from build123d import *

# Parameters (mm, degrees)
F0_W     = 68
F0_H     = 160.5
F1_DEPTH = 10
F2_W     = 46
F2_H     = 17
F3_DEPTH = 25
F4_R     = 5.5
F5_DEPTH = 25
F6_W     = 15
F6_H     = 10
F7_DEPTH = 4
F8_W     = 7
F8_H     = 7
F9_DEPTH = 7


with BuildPart() as f1:
    # F0 (on Front) → F1 (new body)
    with BuildSketch(Plane.XZ):
        with Locations((4.173387, 26.878738)):
            Rectangle(F0_W, F0_H)
    extrude(amount=F1_DEPTH)

    # F2 (on face) → F3 (cut)
    with BuildSketch(Plane.XZ.offset(10)):
        with Locations((-6.826613, 98.628738)):
            Rectangle(F2_W, F2_H)
    extrude(amount=-F3_DEPTH, mode=Mode.SUBTRACT)

    # F4 (on face) → F5 (cut)
    with BuildSketch(Plane.XZ.offset(10)):
        with Locations((27.173387, 98.128738)):
            Circle(F4_R)
    extrude(amount=-F5_DEPTH, mode=Mode.SUBTRACT)

    # F6 (on face) → F7 (cut)
    with BuildSketch(Plane.XZ.offset(10)):
        with Locations((-19.326613, 65.628738)):
            Rectangle(F6_W, F6_H)
    extrude(amount=-F7_DEPTH, mode=Mode.SUBTRACT)

    # F8 (on face) → F9 (join)
    with BuildSketch(Plane.YZ.offset(38.173387)):
        with Locations((-5, -48.371262)):
            Rectangle(F8_W, F8_H)
        with Locations((-5, 67.128738)):
            Rectangle(F8_W, F8_H)
    extrude(amount=F9_DEPTH)


solid = f1.part
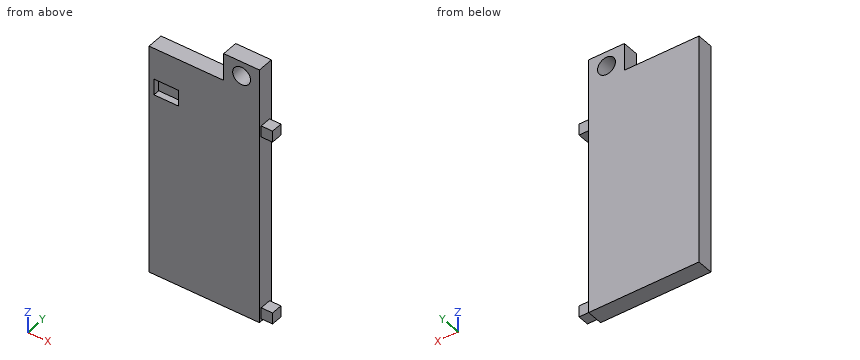
Here's how the part is built. I have some questions about the finished solid (model axes, mm). Coordinates: 2 decimals unless noted, no trailing zeros. Order: outer loops, then holes, each group sorted by start corner. A loop starts at its lowest first (then second) coordinate and runs counter-clockwise, first axis right, second up.
Item 1: For P1, Ø2, axis at x = 42, y = -5, coming from the +Z side; P2, Ø1, axis at y = -3.5, z = 26.5, coming from the +X side; P3, Ø3.5, axis at x = 40.5, z = -48.5, coming from the -Y side, each with a flat end and sliding along its axis, tell me the tip position at first contact or that it passes through.
Result sheet:
P1: stops at z = 70.63
P2: stops at x = 38.17
P3: stops at y = -8.5
Item 2: If we section it at B-B on z = 96: List the corners of the cut face in (x, y) for me, plus the area to 3 significant figures.
Result sheet:
outline: (16.17, -10) - (22.1, -10) - (22.1, 0) - (16.17, 0) - close; (32.24, -10) - (38.17, -10) - (38.17, 0) - (32.24, 0) - close
area: 119 mm2
Item 3: I need wall thicknesses on line 1 (Z direction, x = -16, y = -7); line 2 (Z direction, x = -10.5, y = -6.75); line 3 (X direction, y = -5.75, z = -41). Which ranges of each line are inside material? Lowest first, please.
Result sheet:
line 1: z = -53.37 to 60.63, 70.63 to 90.13
line 2: z = -53.37 to 90.13
line 3: x = -29.83 to 38.17
Item 4: If we section it at A-A on x = -17: List the corners of the cut face in (y, z) for me, plus the area to 4 significant figures.
Result sheet:
outline: (-10, -53.37) - (0, -53.37) - (0, 90.13) - (-10, 90.13) - (-10, 70.63) - (-6, 70.63) - (-6, 60.63) - (-10, 60.63) - close
area: 1,395 mm2
Item 5: If we section it at C-C on x = 27: List the corners of the cut face in (y, z) for me, plus the area to 3 significant figures.
Result sheet:
outline: (-10, -53.37) - (0, -53.37) - (0, 92.63) - (-10, 92.63) - close; (-10, 103.63) - (0, 103.63) - (0, 107.13) - (-10, 107.13) - close
area: 1,500 mm2
Item 6: If we section it at D-D on z = 8: List the corners of the cut face in (x, y) for me.
Result sheet:
outline: (-29.83, -10) - (38.17, -10) - (38.17, 0) - (-29.83, 0) - close
